Check sheet for the modelled part. Datum: model origin and axes. Units: mm. A direction names the side the tool comes from. Coordinates: 2 decimals unless noted, no trailing zeros. Write each loop counter-clockwise with the first axis right and the second up, starting at its lowest first coordinate (ties: lowest second). Pieces come first, ordered by that corner, then holes. Notation, with made-up numbers: (84.5, -12.75) - (119.5, -12.75) arc R25 cw to (119.5, 13.25) - close; hole circle Ø6 at (9.25, -28.75). An arc over 180 degrees is marked (long way). Answer as CSV lines item,"result". Start each with the question number.
from build123d import *

# Parameters (mm, degrees)
F0_W     = 16
F0_H     = 2
F1_DEPTH = 16


with BuildPart() as f1:
    # F0 (on Right) → F1 (new body, symmetric)
    with BuildSketch(Plane.YZ):
        Polygon((10.927957, 0), (-10.927957, 0), (-72.94767, -22.573329), (-72.94767, -25.77426), (75.925268, -25.77426), (75.925268, -11.46078), align=None)
        with Locations((0, -21.77426)):
            Rectangle(F0_W, F0_H, mode=Mode.SUBTRACT)
        Polygon((-27.756056, -9.317461), (-12.720974, -3.845138), (-12.378954, -4.784831), (-12.036934, -5.724524), (-27.072016, -11.196846), align=None, mode=Mode.SUBTRACT)
        with Locations((0, -4)):
            Rectangle(F0_W, F0_H, mode=Mode.SUBTRACT)
        Polygon((-36.939022, -17.874259), (-9.534973, -7.900001), (10.236796, -7.900001), (66.803625, -17.874259), align=None, mode=Mode.SUBTRACT)
    extrude(amount=F1_DEPTH, both=True)


solid = f1.part
(1) Cross-section at B-B on x = -4.5. Record the boundary of the cut face in (y, z).
(2) Tool access check on faces 1 (the face through (0, 0, -20.774)), 2 (the face through (0, 75.925, -19)). Record the directions out of +Z, -Z, +X, -X, +Y, -Y that give a thin tool (end or side, any length) a straight path to the whole face; none if there is none.
(3) Cross-section at D-D on z = -14.5. Record the boundary of the cut face in (x, y).
(4) Release check for a two-part mould opening along Z. For faces 3 (the face through (0.224, 38.124, -12.817)), 4 (the face through (0, -72.948, -24)), 5 (the face through (0.22, 43.88, -5.81)) record: pulls with the +Z half, pulls with the -Z half, needs draft (parallel to the pull), parting line crosses it, or undercut.
(5) Cross-section at C-C on y = 63.5. Record the boundary of the cut face in (x, z), plus the area to 4 significant figures.
(6) Cross-section at A-A on y = -5.5. Record the boundary of the cut face in (x, z), plus the area to 3 significant figures.
(7) Material ranges on probe 1 along Z at (x, y) = (-2.5, -4); probe 2 along Z at (x, y) = (-2, -17); probe 3 along Z at (x, y) = (-5, -16.5), recorded low to high. Write a range as from..to.
Checked values:
1,outline,"(-72.95, -25.77) - (75.93, -25.77) - (75.93, -11.46) - (10.93, 0) - (-10.93, 0) - (-72.95, -22.57) - close; hole (-36.94, -17.87) - (66.8, -17.87) - (10.24, -7.9) - (-9.53, -7.9) - close; hole (-27.76, -9.32) - (-27.07, -11.2) - (-12.04, -5.72) - (-12.72, -3.85) - close; hole (-8, -22.77) - (8, -22.77) - (8, -20.77) - (-8, -20.77) - close; hole (-8, -5) - (8, -5) - (8, -3) - (-8, -3) - close"
2,face 1,"+X, -X"
2,face 2,"+Z, -Z, +X, -X, +Y"
3,outline,"(-16, -50.77) - (16, -50.77) - (16, -27.67) - (-16, -27.67) - close; (-16, 47.67) - (16, 47.67) - (16, 75.93) - (-16, 75.93) - close"
4,face 3,"undercut"
4,face 4,"needs draft"
4,face 5,"pulls with the +Z half"
5,outline,"(-16, -25.77) - (16, -25.77) - (16, -17.87) - (-16, -17.87) - close; (-16, -17.29) - (16, -17.29) - (16, -9.27) - (-16, -9.27) - close"
5,area,"509.5 mm^2"
6,outline,"(-16, -25.77) - (16, -25.77) - (16, -22.77) - (-16, -22.77) - close; (-16, -20.77) - (16, -20.77) - (16, -17.87) - (-16, -17.87) - close; (-16, -7.9) - (16, -7.9) - (16, -5) - (-16, -5) - close; (-16, -3) - (16, -3) - (16, 0) - (-16, 0) - close"
6,area,"378 mm^2"
7,probe 1,"-25.77..-22.77, -20.77..-17.87, -7.9..-5, -3..0"
7,probe 2,"-25.77..-17.87, -10.62..-7.53, -5.4..-2.21"
7,probe 3,"-25.77..-17.87, -10.44..-7.35, -5.22..-2.03"
